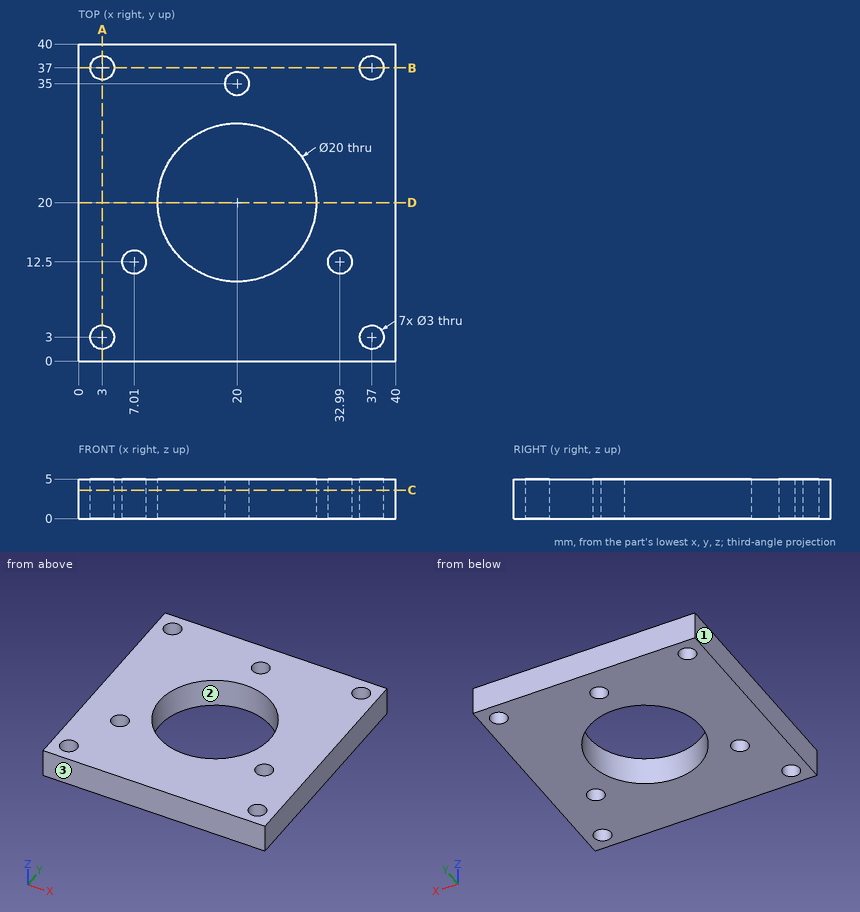
Geometry check sheet. Reference: drawing and pictorial views, mm from the part's lowest x, y, z. Give positions to 0.01 mm unless a question says otherwise; leave off trailing zeros. Write each loop counter-clockwise with the first axis right and the second up, starting at its lowest first coordinate (ties: lowest second). Pieces come first, ordered by that corner, then holes. Notation, with made-up numbers: M -37.5,23.25 L -9.5,23.25 A16 cw -9.5,43.25 Z; hole C 66.5,16 d8. An arc over 180 degrees is marked long. Answer as CSV lines item,"result". Start each with the question number.
Q1. Material ranges on L1, parallel to Y at x = 20, z = 3.35; L2, parallel to Y at x = 37, z = 2.15; L3, parallel to X at y = 36, z = 3.5, recorded low to high.
Q2. Release check for a two-part mould opening along X. For the marked faces 1, 2 and 3 record: pulls with the +X half, pulls with the -X half, needs draft (parallel to the pull), parting line crosses it, or undercut.
Q3. Section check A-A, the plane x = 3. Record the cut outline in (y, z).
Q4. Section check C-C, the plane z = 3.6. Give the number of separate pieces and of enclosed holes in the cut face, then the cut area to 3 significant figures.
Q5. Section check D-D, the plane y = 20. Record the cut outline in (x, z), then the cut area to 3 significant figures.
Geometry says:
1,L1,"0 to 10, 30 to 33.5, 36.5 to 40"
1,L2,"0 to 1.5, 4.5 to 35.5, 38.5 to 40"
1,L3,"0 to 1.88, 4.12 to 18.88, 21.12 to 35.88, 38.12 to 40"
2,face 1,"pulls with the -X half"
2,face 2,"undercut"
2,face 3,"needs draft"
3,outline,"M 0,0 L 1.5,0 L 1.5,5 L 0,5 Z; M 4.5,0 L 35.5,0 L 35.5,5 L 4.5,5 Z; M 38.5,0 L 40,0 L 40,5 L 38.5,5 Z"
4,separate pieces,"1"
4,enclosed holes,"8"
4,area,"1,240 mm^2"
5,outline,"M 0,0 L 10,0 L 10,5 L 0,5 Z; M 30,0 L 40,0 L 40,5 L 30,5 Z"
5,area,"100 mm^2"
